Source: CAD feature listing. Evaluate the final solid. Frame: model axes, mm. Face numbers are marked on the shaded views. A direction names the side the tool comes from. Round coordinates to 2 decimals unless told otherwise and drop trailing zeros. Order: outer loops, then holes, each group sorted by start corner. A loop starts at its lowest first (then second) coordinate and runs counter-clockwise, first axis right, second up. Notation, with made-up numbers: (-13, -16.75) - (25, -16.75) arc R13 ccw to (25, -4.75) - close; hole circle Ø7 at (-39.5, 5). An arc over 180 degrees is marked (long way). Put each result on its own line as item: value. Start each with the question number.
1) Access query for the marked faces 1, 2 and 3. Directions: +Z, -Z, +X, -X, +Y, -Y. A direction counts if a zero-diameter tool reaches every point of the face in a straight line with its end or side. Return the directions, or none.
2) Mould query, pull axis Y, two halves, no side actions, for the marked faces 4, 5, 6 and 7. Classes: +Y half, -Y half, draft (parallel to the pull), parting line (faces both ways), or undercut.
3) Contact query for flat-ended pins moving along their axis: P1, Ø3.5, axis at y = 43.5, z = 8, coming from the -X side; P2, Ø8, axis at y = -24.75, z = 54.75, coming from the +X side; P3, Ø14, axis at x = -28, z = 27.5, coming from the +Y side; P4, Ø6.5, axis at y = 40.5, z = 41.5, coming from the -X side. Output: stop coordinate, or through.
4) Section A-A on z = 40. Output: boundary loops of the cut face in (x, y).
5) Section B-B on y = 0. Output: boundary loops of the cut face in (x, z).
6) Section C-C on x = -19.5. Output: boundary loops of the cut face in (y, z).
7) Line query: probe 1 along Y at (x, z) = (-44, 40); probe 2 along X at (y, z) = (1, 5); probe 3 along X at (y, z) = (37.5, 42). Output: solid intervals per line, ascending. Write a range as [from, to].
8) Section D-D on y = 43.5. Output: boundary loops of the cut face in (x, z).
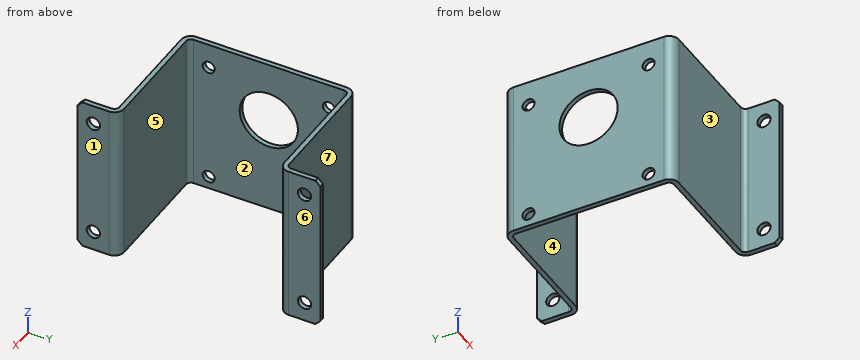
```python
from build123d import *

# Parameters (mm, degrees)
BOSS_EXTRUDE1_DEPTH        = 65
SKETCH2_R                  = 12
CUT_EXTRUDE1_DEPTH         = 99.188594042
F_5_5_5_5_DIAMETER_HOLE1_D = 5.5
F_5_0_5_DIAMETER_HOLE1_D   = 5
CHAMFER1_SIZE              = 2
FILLET1_R                  = 4
FILLET2_R                  = 2


with BuildPart() as part:
    # Sketch1 → Boss-Extrude1 (new body)
    with BuildSketch(Plane.XY):
        Polygon((0, -33), (0, -50), (-2, -50), (-2, -35), (-54, -35), (-54, 35), (-2, 35), (-2, 50), (0, 50), (0, 33), (-52, 33), (-52, -33), align=None)
    extrude(amount=BOSS_EXTRUDE1_DEPTH)

    # Sketch2 → Cut-Extrude1 (cut, through all)
    with BuildSketch(Plane.ZY.offset(54)):
        with Locations(Location((40, 0, 0), (0, 0, 270))):
            Circle(SKETCH2_R)
    extrude(amount=-CUT_EXTRUDE1_DEPTH, mode=Mode.SUBTRACT)

    # Ø5.5 (5.5) Diameter Hole1 (through all)
    with Locations(Plane.ZY.offset(2)):
        with Locations((57, -43.5), (8, -43.5), (57, 43.5), (8, 43.5)):
            Hole(F_5_5_5_5_DIAMETER_HOLE1_D / 2)

    # Ø5.0 (5) Diameter Hole1 (through all)
    with Locations(Plane.ZY.offset(54)):
        with Locations((54.748737342, 24.748737342), (54.748737342, -24.748737342), (5.251262658, -24.748737342), (5.251262658, 24.748737342)):
            Hole(F_5_0_5_DIAMETER_HOLE1_D / 2)

    # Chamfer1
    chamfer1_edges = [part.edges().sort_by_distance(p)[0] for p in [
        (-1, 50, 0),
        (-1, -50, 0),
        (-1, 50, 65),
        (-1, -50, 65),
    ]]
    chamfer(chamfer1_edges, length=CHAMFER1_SIZE)

    # Fillet1
    fillet1_edges = [part.edges().sort_by_distance(p)[0] for p in [
        (-54, -35, 32.5),
        (-54, 35, 32.5),
        (0, 33, 32.5),
        (0, -33, 32.5),
    ]]
    fillet(fillet1_edges, radius=FILLET1_R)

    # Fillet2
    fillet2_edges = [part.edges().sort_by_distance(p)[0] for p in [
        (-2, -35, 32.5),
        (-2, 35, 32.5),
        (-52, 33, 32.5),
        (-52, -33, 32.5),
    ]]
    fillet(fillet2_edges, radius=FILLET2_R)


solid = part.part
```
Answer sheet:
1. face 1: +Z, -Z, +X, +Y, -Y
1. face 2: +Z, -Z, +X
1. face 3: +Z, -Z, -X, -Y
2. face 4: undercut
2. face 5: undercut
2. face 6: draft
2. face 7: +Y half
3. P1: through
3. P2: x = -52
3. P3: y = 35
3. P4: x = -2
4. outline: (-54, -31) arc R4 ccw to (-50, -35) - (-4, -35) arc R2 cw to (-2, -37) - (-2, -50) - (0, -50) - (0, -37) arc R4 ccw to (-4, -33) - (-50, -33) arc R2 cw to (-52, -31) - (-52, -12) - (-54, -12) - close; (-54, 12) - (-52, 12) - (-52, 31) arc R2 cw to (-50, 33) - (-4, 33) arc R4 ccw to (0, 37) - (0, 50) - (-2, 50) - (-2, 37) arc R2 cw to (-4, 35) - (-50, 35) arc R4 ccw to (-54, 31) - close
5. outline: (-54, 0) - (-52, 0) - (-52, 28) - (-54, 28) - close; (-54, 52) - (-52, 52) - (-52, 65) - (-54, 65) - close
6. outline: (-35, 0) - (-33, 0) - (-33, 65) - (-35, 65) - close; (33, 0) - (35, 0) - (35, 65) - (33, 65) - close
7. probe 1: [-35, -33], [33, 35]
7. probe 2: [-54, -52]
7. probe 3: [-2, 0]
8. outline: (-2, 0) - (0, 0) - (0, 5.25) - (-2, 5.25) - close; (-2, 10.75) - (0, 10.75) - (0, 54.25) - (-2, 54.25) - close; (-2, 59.75) - (0, 59.75) - (0, 65) - (-2, 65) - close
